Part model, mm, in its own coordinate system. Face numbers are marked on the shaded views. Round coordinates to 2 decimals unless told otherwise and drop trailing zeros. Order: outer loops, then holes, each group sorted by start corner. A loop starts at its lowest first (then second) coordinate and runs counter-clockwise, first axis right, second up. Notation, with made-up numbers: (65.5, 76) -> (87.5, 76) arc R23 cw to (87.5, 112) -> close; hole circle Ø10 at (40, -10). An arc over 180 degrees is marked (long way). Answer as a JSON object with one key per item and string values. Group by question number.
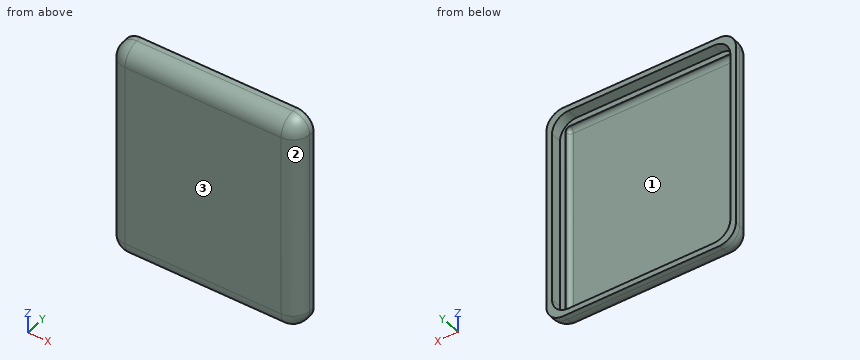
```python
from build123d import *

# Parameters (mm, degrees)
SCHIZZO1_W                   = 34
SCHIZZO1_H                   = 39
ESTRUSIONE_ESTRUSIONE1_DEPTH = 3.95
SCHIZZO2_W                   = 32
SCHIZZO2_H                   = 37
TAGLIO_ESTRUSIONE1_DEPTH     = 2
SCHIZZO3_W                   = 30
SCHIZZO3_H                   = 35
TAGLIO_ESTRUSIONE2_DEPTH     = 0.95
RACCORDO1_R                  = 3
RACCORDO2_R                  = 0.75


with BuildPart() as part:
    # Schizzo1 → Estrusione-Estrusione1 (new body)
    with BuildSketch(Plane(origin=(0, 0, 0), x_dir=(1, 0, 0), z_dir=(0, 1, 0))):
        with Locations((-13.327421164, 1.628483957)):
            Rectangle(SCHIZZO1_W, SCHIZZO1_H)
    extrude(amount=ESTRUSIONE_ESTRUSIONE1_DEPTH)

    # Schizzo2 → Taglio-Estrusione1 (cut)
    with BuildSketch(Plane(origin=(0, 3.95, 0), x_dir=(1, 0, 0), z_dir=(0, 1, 0))):
        with Locations((-13.327421164, 1.628483957)):
            Rectangle(SCHIZZO2_W, SCHIZZO2_H)
    extrude(amount=-TAGLIO_ESTRUSIONE1_DEPTH, mode=Mode.SUBTRACT)

    # Schizzo3 → Taglio-Estrusione2 (cut)
    with BuildSketch(Plane(origin=(0, 1.95, 0), x_dir=(1, 0, 0), z_dir=(0, 1, 0))):
        with Locations((-13.327421164, 1.628483957)):
            Rectangle(SCHIZZO3_W, SCHIZZO3_H)
    extrude(amount=-TAGLIO_ESTRUSIONE2_DEPTH, mode=Mode.SUBTRACT)

    # Raccordo1
    raccordo1_edges = [part.edges().sort_by_distance(p)[0] for p in [
        (-29.327421164, 2.95, 16.871516043),
        (-29.327421164, 2.95, -20.128483957),
        (2.672578836, 2.95, -20.128483957),
        (2.672578836, 2.95, 16.871516043),
        (-13.327421164, 0, -21.128483957),
        (3.672578836, 0, -1.628483957),
        (-13.327421164, 0, 17.871516043),
        (-30.327421164, 0, -1.628483957),
        (-30.327421164, 1.975, -21.128483957),
        (3.672578836, 1.975, -21.128483957),
        (3.672578836, 1.975, 17.871516043),
        (-30.327421164, 1.975, 17.871516043),
    ]]
    fillet(raccordo1_edges, radius=RACCORDO1_R)

    # Raccordo2
    raccordo2_edges = [part.edges().sort_by_distance(p)[0] for p in [
        (-28.327421164, 1, -1.628483957),
        (-28.327421164, 1.475, 15.871516043),
        (-13.327421164, 1, -19.128483957),
        (-28.327421164, 1.475, -19.128483957),
        (1.672578836, 1, -1.628483957),
        (1.672578836, 1.475, -19.128483957),
        (-13.327421164, 1, 15.871516043),
        (1.672578836, 1.475, 15.871516043),
    ]]
    fillet(raccordo2_edges, radius=RACCORDO2_R)


solid = part.part
```
Q1. Band-saw the part on A-A (y = 3.5). List the corners of the cut face in (x, z), plus the area to 3 significant figures.
Q2. Band-saw the part on D-D (y = 0.45). List the corners of the cut face in (x, z).
Q3. Band-saw the part on C-C (z = -8). List the corners of the cut face in (x, y).
Q4. Two-plate mould, pull along X, no slides. Class the marked faces 1, 2 and 3: +X half, -X half, draft (parallel to the pull), parting line (faces both ways), or undercut.
Q5. Band-saw the part on B-B (x = -8). List the corners of the cut face in (y, z).
Q6. Wall check: line 1 (Z direction, x = -6, y = 3.1); line 2 (X direction, y = 3, z = 0.5); line 3 (Y direction, x = -13.5, z = -9). Give the ranges that are in metal, low to high. Write a range as [from, to].
Completed:
{
 "1": {"outline": "(-30.33, -18.13) arc R3 ccw to (-27.33, -21.13) -> (0.67, -21.13) arc R3 ccw to (3.67, -18.13) -> (3.67, 14.87) arc R3 ccw to (0.67, 17.87) -> (-27.33, 17.87) arc R3 ccw to (-30.33, 14.87) -> close; hole (-29.33, -17.13) arc R3 ccw to (-26.33, -20.13) -> (-0.33, -20.13) arc R3 ccw to (2.67, -17.13) -> (2.67, 13.87) arc R3 ccw to (-0.33, 16.87) -> (-26.33, 16.87) arc R3 ccw to (-29.33, 13.87) -> close", "area": "142 mm2"},
 "2": {"outline": "(-28.91, -18.13) arc R1.58 ccw to (-27.33, -19.71) -> (0.67, -19.71) arc R1.58 ccw to (2.25, -18.13) -> (2.25, 14.87) arc R1.58 ccw to (0.67, 16.45) -> (-27.33, 16.45) arc R1.58 ccw to (-28.91, 14.87) -> close"},
 "3": {"outline": "(-30.33, 3) arc R3 ccw to (-27.33, 0) -> (0.67, 0) arc R3 ccw to (3.67, 3) -> (3.67, 3.95) -> (2.67, 3.95) -> (2.67, 1.95) -> (1.67, 1.95) -> (1.67, 1.75) arc R0.75 cw to (0.92, 1) -> (-27.58, 1) arc R0.75 cw to (-28.33, 1.75) -> (-28.33, 1.95) -> (-29.33, 1.95) -> (-29.33, 3.95) -> (-30.33, 3.95) -> close"},
 "4": {"face 1": "undercut", "face 2": "+X half", "face 3": "draft"},
 "5": {"outline": "(0, -18.13) arc R3 ccw to (3, -21.13) -> (3.95, -21.13) -> (3.95, -20.13) -> (1.95, -20.13) -> (1.95, -19.13) -> (1.75, -19.13) arc R0.75 cw to (1, -18.38) -> (1, 15.12) arc R0.75 cw to (1.75, 15.87) -> (1.95, 15.87) -> (1.95, 16.87) -> (3.95, 16.87) -> (3.95, 17.87) -> (3, 17.87) arc R3 ccw to (0, 14.87) -> close"},
 "6": {"line 1": "[-21.13, -20.13], [16.87, 17.87]", "line 2": "[-30.33, -29.33], [2.67, 3.67]", "line 3": "[0, 1]"}
}
